```python
from build123d import *

# Parameters (mm, degrees)
F0_W     = 25
F0_H     = 25
F0_R     = 7
F0_R_2   = 2.925
F1_DEPTH = 35
F2_W     = 25
F2_H     = 22.5
F3_DEPTH = 20
F4_DEPTH = 35.001
F5_R     = 7
F6_DEPTH = 4
F7_R     = 2.5
F8_R     = 3.99999
F9_R     = 0.5


# Not quite as in the source:
# - a fillet or chamfer is up to 0.001 mm smaller than in the source, because OpenCascade refuses the exact size


with BuildPart() as f1:
    # F0 (on Top) → F1 (new body)
    with BuildSketch(Plane.XY):
        Rectangle(F0_W, F0_H)
        with Locations((0, -2)):
            Circle(F0_R, mode=Mode.SUBTRACT)
        with Locations((0, -2)):
            Circle(F0_R)
        with Locations((0, -2)):
            Circle(F0_R_2, mode=Mode.SUBTRACT)
        with Locations((0, -2)):
            Circle(F0_R_2)
    extrude(amount=F1_DEPTH)

    # F2 (on face) → F3 (cut)
    with BuildSketch(Plane.XZ.offset(12.5)):
        with Locations((0, 17.5)):
            Rectangle(F2_W, F2_H)
    extrude(amount=-F3_DEPTH, mode=Mode.SUBTRACT)

    # F0 (on Top) → F4 (cut, through all)
    with BuildSketch(Plane.XY):
        with Locations((0, -2)):
            Circle(F0_R_2)
    extrude(amount=F4_DEPTH, mode=Mode.SUBTRACT)

    # F5 (on face) → F6 (cut)
    with BuildSketch(Plane(origin=(0, 0, 0), x_dir=(1, 0, 0), z_dir=(0, 0, -1))):
        with Locations((0, 2)):
            Circle(F5_R)
    extrude(amount=-F6_DEPTH, mode=Mode.SUBTRACT)

    # F7
    f7_edges = [f1.edges().sort_by_distance(p)[0] for p in [
        (0, 7.5, 6.25),
        (0, 7.5, 28.75),
        (0, 12.5, 35),
        (0, 12.5, 0),
        (0, -12.5, 28.75),
        (0, -12.5, 6.25),
    ]]
    fillet(f7_edges, radius=F7_R)

    # F8 (radius 4 in the source; OpenCascade refuses exactly that, so slightly less here)
    f8_edges = [f1.edges().sort_by_distance(p)[0] for p in [
        (-7, -2, 4),
    ]]
    fillet(f8_edges, radius=F8_R)

    # F9
    f9_edges = [f1.edges().sort_by_distance(p)[0] for p in [
        (-2.925, -2, 35),
        (-2.925, -2, 28.75),
        (-2.925, -2, 6.25),
    ]]
    fillet(f9_edges, radius=F9_R)


solid = f1.part
```
Here's how the part is built. I have some questions about the finished solid (model axes, mm). A direction names the side the tool comes from. Round coordinates to 2 decimals unless told otherwise and drop trailing zeros. Loops run counter-clockwise (first coordinate to the right, second up) from the corner with the lowest first, then second, coordinate; pieces in that order, holes last.
1. If I drill on probe 1 along X at (y, z) = (-2, 4.95) (3 decimals); probe 2 along Y at (x, z) = (0, 32.6) (3 decimals); probe 3 along Z at (x, y) = (-4.25, 4.5), over which ranges is the centre line in solid material (lowest first)?
Answers:
probe 1: x = -12.5 to -2.925, 2.925 to 12.5
probe 2: y = -12.5 to -4.925, 0.925 to 12.498
probe 3: z = 0 to 6.25, 28.75 to 35
2. Suppose I cut it at C-C, the plane z = 5. Please give me the cut outline in (x, y) (3 decimals), and give its area (3 significant figures).
Answers:
outline: (-12.5, -12.165) - (12.5, -12.165) - (12.5, 12.5) - (-12.5, 12.5) - close; hole circle Ø5.85 at (0, -2)
area: 590 mm2
3. Suppose I cut it at D-D, the plane y = -2. Give the number of separate pieces and of enclosed holes in the cut face, and give its area (3 significant figures).
Answers:
separate pieces: 4
enclosed holes: 0
area: 213 mm2
4. Suppose I cut it at A-A, the plane y = 6.5. Please give me the cut outline in (x, z), and give its area (4 significant figures).
Answers:
outline: (-12.5, 0) - (12.5, 0) - (12.5, 6.75) - (-12.5, 6.75) - close; (-12.5, 28.25) - (12.5, 28.25) - (12.5, 35) - (-12.5, 35) - close
area: 337.5 mm2
5. Suppose I cut it at B-B, the plane x = 8. Please give me the cut outline in (y, z).
Answers:
outline: (-12.5, 0) - (10, 0) arc R2.5 ccw to (12.5, 2.5) - (12.5, 32.5) arc R2.5 ccw to (10, 35) - (-12.5, 35) - (-12.5, 31.25) arc R2.5 ccw to (-10, 28.75) - (5, 28.75) arc R2.5 cw to (7.5, 26.25) - (7.5, 8.75) arc R2.5 cw to (5, 6.25) - (-10, 6.25) arc R2.5 ccw to (-12.5, 3.75) - close
6. Thinking about a two-plate mould opening in Z: for faces 1 (the face through (-3, -4, 28.75)), 2 (the face through (0, 12, 1)), 3 (the face through (-0.634, -4.855, 31.838)), which applies, released by +Z, released by -Z, zero draft, split by the parting line, or undercut?
Answers:
face 1: undercut
face 2: released by -Z
face 3: zero draft
7. For faces 4 (the face through (0, -12.5, 33)), 5 (the face through (0.175, 6.748, 28.037)), which set-ups out of +Z, -Z, +X, -X, +Y, -Y let a thin tool reach every point of the face, with its end or its side?
Answers:
face 4: +Z, -Z, +X, -X, -Y
face 5: +X, -X, -Y
8. Will these pins go through, and if not, where does the flat tip stop? pin 1 (3 mm diameter, centred on x = -9, z = 12.5, fed in from -Y); pin 2 (8 mm diameter, centred on x = 2, z = 26.5, fed in from -Y); pin 3 (8.5 mm diameter, centred on x = 0, y = -2, fed in from -Z).
Answers:
pin 1: stops at y = 7.5
pin 2: stops at y = -12.38
pin 3: stops at z = 3.8
